For this review, take the finished solid that the model builds, in its own axes (mm). A direction names the side the tool comes from. Coordinates: 2 decimals unless noted, no trailing zeros. Order: outer loops, then holes, each group sorted by start corner. A loop starts at its lowest first (then second) coordinate and runs counter-clockwise, first axis right, second up.
from build123d import *

# Parameters (mm, degrees)
ESBO_O1_R                = 1.59
RESSALTO_EXTRUS_O1_DEPTH = 15
ESBO_O3_R                = 5
RESSALTO_EXTRUS_O5_DEPTH = 5
ESBO_O8_R                = 1
CORTE_EXTRUS_O1_DEPTH    = 5


with BuildPart() as part:
    # Esboço1 → Ressalto-extrusão1 (new body)
    with BuildSketch(Plane(origin=(0, 0, 0), x_dir=(0, 0, -1), z_dir=(1, 0, 0))):
        Circle(ESBO_O1_R)
    extrude(amount=RESSALTO_EXTRUS_O1_DEPTH)

    # Esboço3 → Ressalto-extrusão5 (add)
    with BuildSketch(Plane.ZY):
        Circle(ESBO_O3_R)
    extrude(amount=RESSALTO_EXTRUS_O5_DEPTH)

    # Esboço8 → Corte-extrusão1 (cut)
    with BuildSketch(Plane.ZY.offset(5)):
        Circle(ESBO_O8_R)
    extrude(amount=-CORTE_EXTRUS_O1_DEPTH, mode=Mode.SUBTRACT)


solid = part.part
1. Clearance check with flat-ended pins moving along their axes: pin 1 Ø1.5 at (y, z) = (3.5, -3) entering from +X; pin 2 Ø4 at (x, z) = (7, -1) entering from +Y; pin 3 Ø6 at (x, y) = (8.5, -3.5) entering from +Z. State where each tip first meets the part, or that it passes through.
Answer below:
pin 1: stops at x = 0
pin 2: stops at y = 1.59
pin 3: stops at z = 1.51
2. Take a section at B-B, the plane x = -1. Give the boundary of the cut face in (y, z).
Answer below:
outline: circle Ø10 at (0, 0); hole circle Ø2 at (0, 0)
3. Machinability: for faces 4 (the face through (15, 0, 0)), 5 (the face through (-3, -1, 0)), 6 (the face through (0, 0, 2)), which of the approach directions +Z, -Z, +X, -X, +Y, -Y give a long, thin tool a straight path to every point of the face, cutting with its end or side? Answer none if there is none.
Answer below:
face 4: +Z, -Z, +X, +Y, -Y
face 5: -X
face 6: +X
4. Take a section at C-C, the plane y = 0.5. Give the boundary of the cut face in (x, z).
Answer below:
outline: (-5, -4.97) - (0, -4.97) - (0, -1.51) - (15, -1.51) - (15, 1.51) - (0, 1.51) - (0, 4.97) - (-5, 4.97) - (-5, 0.87) - (0, 0.87) - (0, -0.87) - (-5, -0.87) - close
5. Take a section at A-A, the plane z = 0. Give the boundary of the cut face in (x, y).
Answer below:
outline: (-5, -5) - (0, -5) - (0, -1.59) - (15, -1.59) - (15, 1.59) - (0, 1.59) - (0, 5) - (-5, 5) - (-5, 1) - (0, 1) - (0, -1) - (-5, -1) - close
6. To check wall thickness, follow L1, parallel to Y at x = -1.7, z = 0; L2, parallel to X at y = 0.5, z = 3.25; L3, parallel to X at y = -0.5, z = 0.25. State the ranges of each line that lie inside material, in increasing order.
Answer below:
L1: y = -5 to -1, 1 to 5
L2: x = -5 to 0
L3: x = 0 to 15
7. Take a section at D-D, the plane x = 13.25. Give the boundary of the cut face in (y, z).
Answer below:
outline: circle Ø3.18 at (0, 0)
8. The part is to be moulded in two halves that separate along Y. For faces 1 (the face through (-5, 1.2, -0.1)), 2 (the face through (-2.46, -4.88, -1.08)), 3 (the face through (0, 0, 0)), say which applies: +Y half, -Y half, draft (parallel to the pull), parting line (faces both ways), or undercut.
Answer below:
face 1: draft
face 2: parting line
face 3: undercut
